Verification items for this drawing (mm, ordinates from the low corner). Round coordinates to 2 decimals unless told otherwise and drop trailing zeros. Write each loop counter-clockwise with the first axis right and the second up, starting at its lowest first coordinate (ties: lowest second). Pieces come first, ordered by that corner, then holes. Notation, with made-up numbers: M 4,1 L 42,1 A18 cw 42,19 Z; hole C 1.25,6.5 d5. An arc over 180 degrees is marked long. Write each question's results on one line, items separated by ' | '.
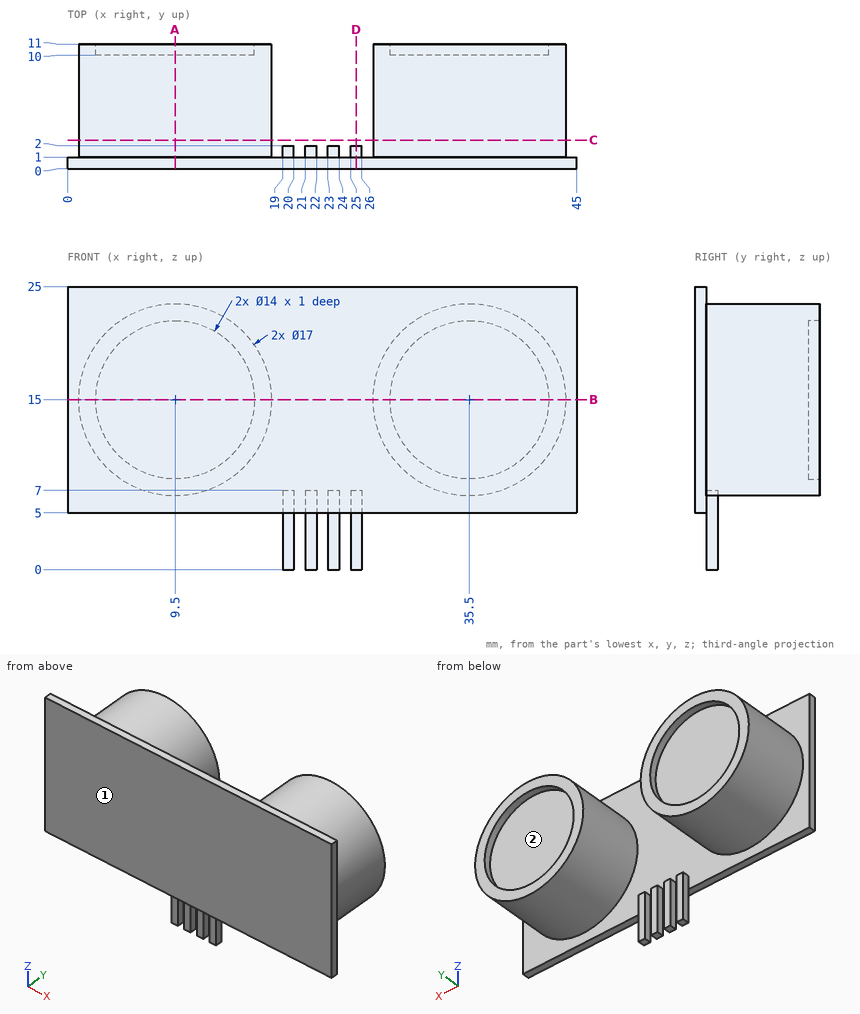
1) Sectioned sample at A-A, the plane x = 9.5. Record the cut outline in (y, z).
Calculated:
outline: M 0,5 L 1,5 L 1,6.5 L 11,6.5 L 11,8 L 10,8 L 10,22 L 11,22 L 11,23.5 L 1,23.5 L 1,25 L 0,25 Z
2) Sectioned sample at C-C, the plane y = 2.5. Record the cut outline in (x, z), and give its area (3 significant figures).
Calculated:
outline: C 9.5,15 d17; C 35.5,15 d17 | area: 454 mm²
3) Draft check along X on the marked faces 1 and 2. Enter one of: pulls with the +X half, pulls with the -X half, needs draft (parallel to the pull), parting line crosses it, or undercut.
Calculated:
face 1: needs draft | face 2: undercut
4) Sectioned sample at B-B, the plane z = 15. Record the cut outline in (x, y).
Calculated:
outline: M 0,0 L 45,0 L 45,1 L 44,1 L 44,11 L 42.5,11 L 42.5,10 L 28.5,10 L 28.5,11 L 27,11 L 27,1 L 18,1 L 18,11 L 16.5,11 L 16.5,10 L 2.5,10 L 2.5,11 L 1,11 L 1,1 L 0,1 Z
5) Material ranges on line 1 (X direction, y = 10.65, z = 15); line 2 (Y direction, x = 31.5, z = 14.75); line 3 (X direction, y = 8.5, z = 17), recorded low to high. Write a range as [from, to].
Calculated:
line 1: x = [1, 2.5], [16.5, 18], [27, 28.5], [42.5, 44] | line 2: y = [0, 10] | line 3: x = [1.24, 17.76], [27.24, 43.76]
6) Sectioned sample at D-D, the plane x = 25.5. Record the cut outline in (y, z).
Calculated:
outline: M 0,5 L 1,5 L 1,0 L 2,0 L 2,7 L 1,7 L 1,25 L 0,25 Z
7) Depth check by flat-ended pin: P1, Ø0.8, axis at x = 25.5, z = 4.5, coming from the +Y side; P2, Ø0.8, axis at y = 1.5, z = 2, coming from the +X side; P3, Ø2, axis at y = 6, z = 16.5, coming from the -X side. Enter the tip coordinate at first touch or a pass-through.
Calculated:
P1: stops at y = 2 | P2: stops at x = 26 | P3: stops at x = 1.01
